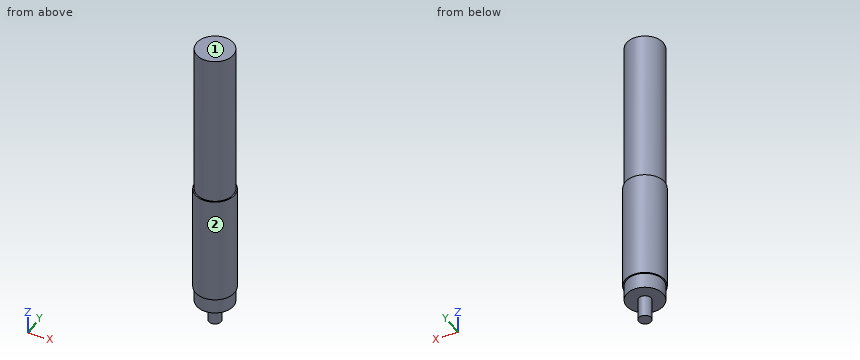
Autodesk Inventor part; units mm, degrees
ref_plane "YZ Plane" through (0, 0, 0) normal (1, 0, 0) x (0, 1, 0)
ref_plane "XZ Plane" through (0, 0, 0) normal (0, 1, 0) x (-1, 0, 0)
ref_plane "XY Plane" through (0, 0, 0) normal (0, 0, 1) x (1, 0, 0)
sketch "Sketch1" plane through (0, 0, 0) normal (0, 1, 0) x (-1, 0, 0)
  line L0 (0, 0) -> (-5.9, 0)
  line L1 (-5.9, 0) -> (-5.9, -50)
  line L2 (-5.9, -50) -> (-6.3, -50)
  line L3 (-6.3, -50) -> (-6.3, -85)
  line L4 (-6.3, -85) -> (-5.9, -85)
  line L5 (-5.9, -85) -> (-5.9, -90)
  line L6 (-5.9, -90) -> (-2, -90)
  line L7 (-2, -90) -> (-2, -97)
  line L8 (-2, -97) -> (0, -97)
  line L9 (0, -97) -> (0, 0)
  dimension "d1" = 5.9
  dimension "d2" = 50
  dimension "d3" = 7
  dimension "d4" = 5
  dimension "d5" = 35
  dimension "d7" = 6.3
  dimension "d8" = 2
revolve "Revolution1" add sketch "Sketch1" angle 360 about axis through (0, 0, -97) along (0, 0, 1)
thread "Thread1"
properties part number "holdingRod"
The model under review builds one solid part; all positions refer to its coordinate system, in mm. Face numbers are marked on the shaded views. Give positions to 0.01 mm unless a question says otherwise; leave off trailing zeros. Loops run counter-clockwise (first coordinate to the right, second up) from the corner with the lowest first, then second, coordinate; pieces in that order, holes last. Notation, with made-up numbers: (10.5, -14) -> (65.5, -14) arc R17 cw to (65.5, -10) -> close; hole circle Ø7 at (3, -4). An arc over 180 degrees is marked (long way). Write each question's results on one line, items separated by ' | '.
1) Draft analysis for pull direction Z (two halves, no side actions). For the marked faces 1 and 2, state which applies: pulls with the +Z half, pulls with the -Z half, needs draft (parallel to the pull), parting line crosses it, or undercut.
Conclusion:
face 1: pulls with the +Z half | face 2: needs draft
2) For line 1 along Z through (x, y) = (-5.5, 1.75); line 2 along X through (y, z) = (0.5, -62); line 3 along X through (y, z) = (2.25, -10), list the stretches that pass through material, from the lowest coordinate up. Write a range as from..to.
Conclusion:
line 1: z = -90..0 | line 2: x = -6.28..6.28 | line 3: x = -5.45..5.45
3) Take a section at C-C, the plane z = -71. Give the boundary of the cut face in (x, y).
Conclusion:
outline: circle Ø12.6 at (0, 0)
4) Insertion check: pin 1 Ø1.5 at (y, z) = (2.5, -31) entering from -X; pin 2 Ø3 at (y, z) = (-4.5, -18.5) entering from +X; pin 3 Ø3 at (x, y) = (-0.5, 4.5) entering from -Z. Each pin has a flat end and moves straight along its axis. Give the tip position at first contact, or say it passes through.
Conclusion:
pin 1: stops at x = -5.63 | pin 2: stops at x = 5.08 | pin 3: stops at z = -90
5) Take a section at D-D, the plane x = 4.25. Give the boundary of the cut face in (y, z).
Conclusion:
outline: (-4.65, -85) -> (-4.09, -85) -> (-4.09, -90) -> (4.09, -90) -> (4.09, -85) -> (4.65, -85) -> (4.65, -50) -> (4.09, -50) -> (4.09, 0) -> (-4.09, 0) -> (-4.09, -50) -> (-4.65, -50) -> close
6) Take a section at A-A, the plane y = 0. Give the boundary of the cut face in (x, z), plus the area to 3 significant figures.
Conclusion:
outline: (-6.3, -85) -> (-5.9, -85) -> (-5.9, -90) -> (-2, -90) -> (-2, -97) -> (2, -97) -> (2, -90) -> (5.9, -90) -> (5.9, -85) -> (6.3, -85) -> (6.3, -50) -> (5.9, -50) -> (5.9, 0) -> (-5.9, 0) -> (-5.9, -50) -> (-6.3, -50) -> close | area: 1,120 mm^2
